Build history of the part. All positions in model axes, mm. A direction names the side the tool comes from. Coordinates: 2 decimals unless noted, no trailing zeros. Loops run counter-clockwise (first coordinate to the right, second up) from the corner with the lowest first, then second, coordinate; pieces in that order, holes last.
Item 1: Cut at C-C (x = 549.5). List the corners of the cut face in (y, z), and give its area (3 significant figures).
Item 2: 3-axis set-ups, long thin cutter, end or side, ignore diameter. For faces 5 (the face through (16, 0, 1095)), 6 (the face through (972, -242, 862)): which of +Z, -Z, +X, -X, +Y, -Y reach the whole face in a straight line?
Item 3: Drill centre lines: line 1 along X through (y, z) = (-87, 340); line 2 along Z through (x, y) = (470, -429); line 3 along X through (y, z) = (-496.5, 349). Where is each one in solid material? Low to high.
Item 4: Cut at A-A (z = 562). List the corners of the cut face in (x, y), and give its area (3 significant figures).
Item 5: Cut at B-B (y = -192). List the corners of the cut face in (x, z).
Item 6: Flat gauge pins, fed straight in: pin 1 (5 mm diameter, centred on x = 666.5, y = -442.5, fed in from +Z); pin 2 (1.5 mm diameter, centred on x = 508, y = -207, fed in from -Z). Where does each tip first touch, or does it go through?
Item 7: Mould opens along X. For faces 1 (the face through (0, -291, 1105)), 2 (the face through (990, -242, 1075)), 3 (the face through (502, -242, 1718)), 4 (the face through (972, -242, 1952)) say: released by +X, released by -X, zero draft, split by the parting line, or undercut.
Item 8: Cut at D-D (y = -524.5). List the corners of the cut face in (x, z), and give its area (3 significant figures).
from build123d import *

# Parameters (mm, degrees)
F1_DEPTH = 490
F2_W     = 100
F2_H     = 2180
F3_DEPTH = 18


with BuildPart() as f1:
    # F0 (on Front) → F1 (new body)
    with BuildSketch(Plane.XZ):
        Polygon((0, 2180), (0, 0), (18, 0), (18, 1700), (972, 1700), (972, 0), (990, 0), (990, 2180), (972, 2180), (972, 2162), (972, 1718), (18, 1718), (18, 2162), (18, 2180), align=None)
    extrude(amount=F1_DEPTH)

    # F2 (on face) → F3 (join)
    with BuildSketch(Plane(origin=(0, 0, 0), x_dir=(0, -1, 0), z_dir=(-1, 0, 0))):
        with Locations((540, 1090)):
            Rectangle(F2_W, F2_H)
    extrude(amount=-F3_DEPTH)


solid = f1.part
Filled sheet:
1. outline: (-490, 1700) - (0, 1700) - (0, 1718) - (-490, 1718) - close
1. area: 8,820 mm2
2. face 5: +Z, -Z, +X, -X, +Y
2. face 6: -Z, +Y, -Y
3. line 1: x = 0 to 18, 972 to 990
3. line 2: z = 1700 to 1718
3. line 3: x = 0 to 18
4. outline: (0, -590) - (18, -590) - (18, 0) - (0, 0) - close; (972, -490) - (990, -490) - (990, 0) - (972, 0) - close
4. area: 19,400 mm2
5. outline: (0, 0) - (18, 0) - (18, 1700) - (972, 1700) - (972, 0) - (990, 0) - (990, 2180) - (972, 2180) - (972, 1718) - (18, 1718) - (18, 2180) - (0, 2180) - close
6. pin 1: stops at z = 1718
6. pin 2: stops at z = 1700
7. face 1: released by -X
7. face 2: released by +X
7. face 3: undercut
7. face 4: undercut
8. outline: (0, 0) - (18, 0) - (18, 2180) - (0, 2180) - close
8. area: 39,200 mm2
